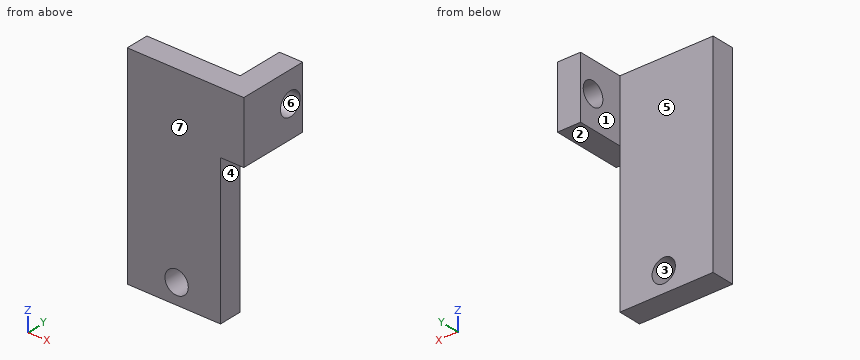
```python
from build123d import *

# Parameters (mm, degrees)
CROQUIS1_W              = 12
CROQUIS1_H              = 27
CROQUIS1_R              = 1.5
SALIENTE_EXTRUIR2_DEPTH = 3
CROQUIS6_W              = 8
CROQUIS6_H              = 9
CROQUIS6_R              = 1.5
SALIENTE_EXTRUIR4_DEPTH = 3
ESCALA1_SCALE           = 7


with BuildPart() as part:
    # Croquis1 → Saliente-Extruir2 (new body)
    with BuildSketch(Plane(origin=(0, 0, 0), x_dir=(1, 0, 0), z_dir=(0, 1, 0))):
        with Locations((6, 13.5)):
            Rectangle(CROQUIS1_W, CROQUIS1_H)
        with Locations((6.352695101, 24.378103836)):
            Circle(CROQUIS1_R, mode=Mode.SUBTRACT)
    extrude(amount=SALIENTE_EXTRUIR2_DEPTH)

    # Croquis6 → Saliente-Extruir4 (add)
    with BuildSketch(Plane(origin=(12, 0, 0), x_dir=(0, 0, -1), z_dir=(1, 0, 0))):
        with Locations((4, 4.5)):
            Rectangle(CROQUIS6_W, CROQUIS6_H)
        with Locations((3.905842021, 7.100326765)):
            Circle(CROQUIS6_R, mode=Mode.SUBTRACT)
    extrude(amount=SALIENTE_EXTRUIR4_DEPTH)


with BuildPart() as part_1:
    # Escala1: scaled about (7.268760736, 1.961981653, -11.685014046)
    add(part.part.scale(ESCALA1_SCALE).moved(Location((-43.612564416, -11.771889918, 70.110084276))))


solid = part_1.part
```
Geometry: final body of the model. Coordinates: model frame, mm. Face numbers are marked on the shaded views. A direction names the side the tool comes from. Coordinates: 2 decimals unless noted, no trailing zeros. Order: outer loops, then holes, each group sorted by start corner. A loop starts at its lowest first (then second) coordinate and runs counter-clockwise, first axis right, second up. Notation, with made-up numbers: (57, 32) -> (88, 32) arc R24 ccw to (88, 63) -> close; hole circle Ø5 at (1, 51). An arc over 180 degrees is marked (long way). Write each question's results on one line, items separated by ' | '. Start each with the question number.
1) Cut plane B-B, the plane y = -3. Output: boundary loops of the cut face in (x, z), and give its area (3 significant figures).
2) Material intervals for line 1 along Y through (x, z) = (-27, 1); line 2 along Z through (x, y) = (42, 10); line 3 along Z through (x, y) = (53.5, 29), sorted ascending.
3) Cut plane A-A, the plane z = -92.5. Output: boundary loops of the cut face in (x, y), and give its area (3 significant figures).
4) First-contact query: pin 1 (10.5 mm diameter, centred on x = 52.5, y = 6, fed in from -Z); pin 2 (6.5 mm diameter, centred on y = -2, z = -22, fed in from +X). Flat tips, straight axial feed; report the tip coordinate or a pass-through.
5) Cut plane D-D, the plane x = 45. Output: boundary loops of the cut face in (y, z).
6) Mould query, pull axis Y, two halves, no side actions, for the marked faces 4, 5, 6 and 7. Classes: released by +Y, released by -Y, zero draft, split by the parting line, or undercut.
7) Set-up query: the marked faces 1, 2 and 3. Return all of +Z, -Z, +X, -X, +Y, -Y with unobstructed straight access to the full face (end or side cutting, diameter ignored); none if empty.
8) Cut plane C-C, the plane x = 4.5. Output: boundary loops of the cut face in (y, z), and give its area (3 significant figures).
Checks:
1) outline: (-43.61, -118.89) -> (40.39, -118.89) -> (40.39, 14.11) -> (61.39, 14.11) -> (61.39, 70.11) -> (-43.61, 70.11) -> close; hole circle Ø21 at (0.86, -100.54) | area: 16,700 mm^2
2) line 1: -11.77 to 9.23 | line 2: 14.11 to 70.11 | line 3: 14.11 to 37.25, 48.29 to 70.11
3) outline: (-43.61, -11.77) -> (-5.9, -11.77) -> (-5.9, 9.23) -> (-43.61, 9.23) -> close; (7.61, -11.77) -> (40.39, -11.77) -> (40.39, 9.23) -> (7.61, 9.23) -> close | area: 1,480 mm^2
4) pin 1: z = 14.11 | pin 2: x = 40.39
5) outline: (-11.77, 14.11) -> (51.23, 14.11) -> (51.23, 70.11) -> (-11.77, 70.11) -> close; hole circle Ø21 at (37.93, 42.77)
6) face 4: zero draft | face 5: released by +Y | face 6: undercut | face 7: released by -Y
7) face 1: +Z, -Z, -X, +Y | face 2: -Z, +X, +Y, -Y | face 3: +Y, -Y
8) outline: (-11.77, -118.89) -> (9.23, -118.89) -> (9.23, -110.38) -> (-11.77, -110.38) -> close; (-11.77, -90.69) -> (9.23, -90.69) -> (9.23, 70.11) -> (-11.77, 70.11) -> close | area: 3,560 mm^2
